For this review, take the finished solid that the model builds, in its own axes (mm). A direction names the side the tool comes from. Coordinates: 2 decimals unless noted, no trailing zeros. Loops run counter-clockwise (first coordinate to the right, second up) from the corner with the lowest first, then second, coordinate; pieces in that order, holes last.
1. Machinability: for faces 1 (the face through (31.43, -2.68, -25.52)), 2 (the face through (-31.37, -2.68, -25.58)), 3 (the face through (-0.762, 0, 31)), 4 (the face through (28.448, 10, 30)), which of the approach directions +Z, -Z, +X, -X, +Y, -Y give a long, thin tool a straight path to every point of the face, cutting with its end or side? Answer none if there is none.
2. Take a section at C-C, the plane x = 14. State the section outline as (y, z) points, then the cut area to 3 significant figures.
3. Take a section at A-A, the plane y = 9. State the section outline as (x, z) points (3 decimals), then the cut area to 3 significant figures.
4. To check wall thickness, follow probe 1 along Y at (x, z) = (19.5, -3.5); probe 2 along X at (y, z) = (3.5, 34); probe 3 along X at (y, z) = (0.5, -13). State the ranges of each line that lie inside material, in increasing order.
5. Take a section at D-D, the plane z = 0. State the section outline as (x, y) points, then the cut area to 3 significant figures.
6. Take a section at B-B, the plane z = -13.97. State the section outline as (x, y) points, then the cut area to 3 significant figures.
7. Clearance check with flat-ended pins moving along their axes: P1, Ø3, axis at x = -20.5, z = 32, coming from the -Y side; P2, Ø5, axis at x = 19.812, z = -39.37, coming from the +Y side; P3, Ø2.5, axis at y = 10.5, z = 30.5, coming from the -X side; P4, Ø2.5, axis at y = 10, z = 31, coming from the +X side. State where each tip first meets the part, or that it passes through.
```python
from build123d import *

# Parameters (mm, degrees)
F0_W          = 65.024
F0_H          = 53.34
F1_DEPTH      = 12.7
F1_DEPTH_BACK = 12.7
F2_W          = 31.75
F2_H          = 12.7
F3_DEPTH      = 25.4
F4_W          = 25.4
F4_H          = 6.35
F5_DEPTH      = 5.08
F7_W          = 12.7
F7_H          = 5.08
F8_ANGLE      = 180
F9_R          = 3.175
F10_DEPTH     = 25.4
F11_W         = 5.08
F11_H         = 25.4
F12_DEPTH     = 6.35
F13_W         = 5.08
F13_H         = 12.7
F15_R         = 3.175
F16_DEPTH     = 25.4
F17_W         = 25.4
F17_H         = 5.08
F18_DEPTH     = 6.35
F19_W         = 12.7
F19_H         = 5.08
F21_R         = 3.175
F22_DEPTH     = 25.4
F23_R         = 3.81
F24_R         = 6.6929
F24_R_2       = 2.54
F25_DEPTH     = 12.7
F26_R         = 3.81
F27_DEPTH     = 38.1


with BuildPart() as f1:
    # F0 (on Front) → F1 (new body, two sides)
    with BuildSketch(Plane.XZ) as f1_sk:
        Rectangle(F0_W, F0_H)
    extrude(amount=F1_DEPTH)
    extrude(f1_sk.sketch, amount=-F1_DEPTH_BACK)

    # F2 (on face) → F3 (join)
    with BuildSketch(Plane.XZ.offset(12.7)):
        with Locations((-16.637, 33.02)):
            Rectangle(F2_W, F2_H)
    extrude(amount=-F3_DEPTH)

    # F4 (on face) → F5 (join)
    with BuildSketch(Plane(origin=(0, 12.7, 0), x_dir=(-1, 0, 0), z_dir=(0, 1, 0))):
        with Locations((-15.748, 29.845)):
            Rectangle(F4_W, F4_H)
    extrude(amount=-F5_DEPTH)

    # F7 (on face) → F8 (revolve)
    with BuildSketch(Plane.XY.offset(33.02)):
        with Locations((22.098, 10.16)):
            Rectangle(F7_W, F7_H)
    revolve(axis=Axis((15.748, 10.16, 33.02), (0, -1, 0)), revolution_arc=F8_ANGLE)

    # F9 (on face) → F10 (cut)
    with BuildSketch(Plane(origin=(0, 12.7, 0), x_dir=(-1, 0, 0), z_dir=(0, 1, 0))):
        with Locations((-15.748, 39.37)):
            Circle(F9_R)
    extrude(amount=-F10_DEPTH, mode=Mode.SUBTRACT)

    # F11 (on face) → F12 (join)
    with BuildSketch(Plane(origin=(-32.512, 0, 0), x_dir=(0, -1, 0), z_dir=(-1, 0, 0))):
        with Locations((-10.16, -13.97)):
            Rectangle(F11_W, F11_H)
    extrude(amount=F12_DEPTH)

    # F13 (on face) → F14 (revolve)
    with BuildSketch(Plane(origin=(-38.862, 0, 0), x_dir=(0, -1, 0), z_dir=(-1, 0, 0))):
        with Locations((-10.16, -7.62)):
            Rectangle(F13_W, F13_H)
    revolve(axis=Axis((-38.862, 10.16, -13.97), (0, -1, 0)))

    # F15 (on face) → F16 (cut)
    with BuildSketch(Plane.XZ.offset(-7.62)):
        with Locations((-45.212, -13.97)):
            Circle(F15_R)
    extrude(amount=-F16_DEPTH, mode=Mode.SUBTRACT)

    # F17 (on face) → F18 (join)
    with BuildSketch(Plane(origin=(0, 0, -26.67), x_dir=(1, 0, 0), z_dir=(0, 0, -1))):
        with Locations((19.812, -10.16)):
            Rectangle(F17_W, F17_H)
    extrude(amount=F18_DEPTH)

    # F19 (on face) → F20 (revolve)
    with BuildSketch(Plane(origin=(0, 0, -33.02), x_dir=(1, 0, 0), z_dir=(0, 0, -1))):
        with Locations((13.462, -10.16)):
            Rectangle(F19_W, F19_H)
    revolve(axis=Axis((19.812, 10.16, -33.02), (0, -1, 0)))

    # F21 (on face) → F22 (cut)
    with BuildSketch(Plane.XZ.offset(-7.62)):
        with Locations((19.812, -39.37)):
            Circle(F21_R)
    extrude(amount=-F22_DEPTH, mode=Mode.SUBTRACT)

    # F23
    f23_edges = [f1.edges().sort_by_distance(p)[0] for p in [
        (-0.762, 0, 39.37),
        (-32.512, 0, 39.37),
        (32.512, 0, 26.67),
        (32.512, -2.54, -26.67),
        (-32.512, -2.54, -26.67),
    ]]
    fillet(f23_edges, radius=F23_R)

    # F24 (on face) → F25 (join)
    with BuildSketch(Plane.XZ.offset(12.7)):
        Circle(F24_R)
        Circle(F24_R_2, mode=Mode.SUBTRACT)
    extrude(amount=F25_DEPTH)

    # F26 (on face) → F27 (join)
    with BuildSketch(Plane.XZ.offset(12.7)):
        Circle(F26_R)
    extrude(amount=F27_DEPTH)


solid = f1.part
```
Results list:
1. face 1: -Z, +X, -Y
1. face 2: -Z, -X, -Y
1. face 3: +Z, +Y, -Y
1. face 4: +Z, +X, +Y, -Y
2. outline: (-12.7, -26.67) - (7.62, -26.67) - (7.62, -44.31) - (12.7, -44.31) - (12.7, 36.72) - (7.62, 36.72) - (7.62, 26.67) - (-12.7, 26.67) - close; (7.62, 42.02) - (12.7, 42.02) - (12.7, 45.6) - (7.62, 45.6) - close
2. area: 1,510 mm2
3. outline: (-38.862, -26.67) - (7.112, -26.67) - (7.112, -33.02) arc R12.7 ccw to (32.512, -33.02) - (32.512, 22.86) arc R3.81 ccw to (28.702, 26.67) - (28.448, 26.67) - (28.448, 33.02) arc R12.7 ccw to (3.048, 33.02) - (3.048, 26.67) - (-0.762, 26.67) - (-0.762, 35.56) arc R3.81 ccw to (-4.572, 39.37) - (-28.702, 39.37) arc R3.81 ccw to (-32.512, 35.56) - (-32.512, -1.27) - (-38.862, -1.27) arc R12.7 ccw to start; hole circle Ø6.35 at (-45.212, -13.97); hole circle Ø6.35 at (15.748, 39.37); hole circle Ø6.35 at (19.812, -39.37)
3. area: 5,010 mm2
4. probe 1: y = -12.7 to 12.7
4. probe 2: x = -32.51 to -0.76
4. probe 3: x = -32.51 to 32.51
5. outline: (-32.51, -12.7) - (-6.69, -12.7) - (-6.69, -25.4) - (-3.81, -25.4) - (-3.81, -50.8) - (3.81, -50.8) - (3.81, -25.4) - (6.69, -25.4) - (6.69, -12.7) - (32.51, -12.7) - (32.51, 12.7) - (-32.51, 12.7) - close
5. area: 2,020 mm2
6. outline: (-51.56, 7.62) - (-48.39, 7.62) - (-48.39, 12.7) - (-51.56, 12.7) - close; (-42.04, 7.62) - (-32.51, 7.62) - (-32.51, -12.7) - (32.51, -12.7) - (32.51, 12.7) - (-42.04, 12.7) - close
6. area: 1,720 mm2
7. P1: stops at y = -12.7
7. P2: passes through
7. P3: stops at x = -32.51
7. P4: stops at x = 28.45
